Can you work these out from the model? Positions are in its coordinate system, mm. Round coordinates to 2 decimals unless told otherwise and drop trailing zeros. Loops run counter-clockwise (first coordinate to the right, second up) from the corner with the lowest first, then second, coordinate; pieces in that order, holes last.
```python
from build123d import *

# Parameters (mm, degrees)
SKETCH1_R             = 12.7
SKETCH1_R_2           = 2.5
BOSS_EXTRUDE1_DEPTH   = 8.89
F_2_56_TAPPED_HOLE1_D = 1.778
SKETCH6_W             = 1.1303
SKETCH6_H             = 12.7


with BuildPart() as part:
    # Sketch1 → Boss-Extrude1 (new body)
    with BuildSketch(Plane.XY):
        Circle(SKETCH1_R)
        Circle(SKETCH1_R_2, mode=Mode.SUBTRACT)
    extrude(amount=BOSS_EXTRUDE1_DEPTH)

    # #2-56 Tapped Hole1 (through all)
    with Locations(Plane.XY.offset(8.89)):
        with Locations((-8.255, 6.35), (8.255, 6.35), (8.255, -6.35), (-8.255, -6.35)):
            Hole(F_2_56_TAPPED_HOLE1_D / 2)

    # Sketch6 → #4-40 Tapped Hole1 (revolve, cut)
    with BuildSketch(Plane(origin=(0, 0, 4.445), x_dir=(0, 0, -1), z_dir=(1, 0, 0))):
        with Locations((0.56515, 6.35)):
            Rectangle(SKETCH6_W, SKETCH6_H)
    revolve(axis=Axis((0, -6.35, 4.445), (0, 1, 0)), mode=Mode.SUBTRACT)


solid = part.part
```
(1) If I drill on line 1 (Y direction, x = 0, z = 7); line 2 (X direction, y = 6.5, z = 3.25); line 3 (X direction, y = -6, z = 1.75), over which ranges is the centre line in solid material (lowest first)?
(2) We'd pull the mould along Y, two halves only. Please class faces 1 (the cylindrical face through (0.69, 7.54, 5.34)), 2 (the cylindrical face through (-2.75, -12.4, 4.38)), 3 (the cylindrical face through (-0.54, -2.44, 4.38)): released by +Y, released by -Y, zero draft, split by the parting line, or undercut.
(3) Suppose I cut it at B-B (y = 0). Write out the boundary of the cut face in (x, z).
(4) Suppose I cut it at C-C (y = -6.35). Write out the boundary of the cut face in (x, z), then the cut area to 3 significant figures.
(5) Suppose I cut it at D-D (z = 2). Write out the boundary of the cut face in (x, y) (3 decimals).
(6) For pin 1 (1.5 mm diameter, centred on y = 1.5, z = 5.5, fed in from -X); pin 2 (1 mm diameter, centred on x = 6, z = 4.5, fed in from -Y); pin 3 (4 mm diameter, centred on x = 3, z = 1, fed in from -Y), each with a flat end and sliding along its axis, tell me the tip position at first contact or that it passes through.
(7) Suppose I cut it at A-A (x = 0). Write out the boundary of the cut face in (y, z), then the cut area to 3 significant figures.
Check result:
1. line 1: y = -12.7 to -2.5, 2.5 to 12.7
1. line 2: x = -10.91 to -9.13, -7.38 to 7.38, 9.13 to 10.91
1. line 3: x = -11.19 to -9.07, -7.44 to 7.44, 9.07 to 11.19
2. face 1: zero draft
2. face 2: split by the parting line
2. face 3: undercut
3. outline: (-12.7, 0) - (-2.5, 0) - (-2.5, 8.89) - (-12.7, 8.89) - close; (2.5, 0) - (12.7, 0) - (12.7, 8.89) - (2.5, 8.89) - close
4. outline: (-11, 0) - (-9.14, 0) - (-9.14, 8.89) - (-11, 8.89) - close; (-7.37, 0) - (7.37, 0) - (7.37, 8.89) - (-7.37, 8.89) - close; (9.14, 0) - (11, 0) - (11, 8.89) - (9.14, 8.89) - close
4. area: 164 mm2
5. outline: circle Ø25.4 at (0, 0); hole circle Ø1.778 at (-8.255, -6.35); hole circle Ø1.778 at (-8.255, 6.35); hole circle Ø5 at (0, 0); hole circle Ø1.778 at (8.255, -6.35); hole circle Ø1.778 at (8.255, 6.35)
6. pin 1: stops at x = -12.68
6. pin 2: stops at y = -11.45
6. pin 3: stops at y = -12.66
7. outline: (-12.7, 0) - (-2.5, 0) - (-2.5, 8.89) - (-12.7, 8.89) - close; (2.5, 0) - (12.7, 0) - (12.7, 3.31) - (2.5, 3.31) - close; (2.5, 5.58) - (12.7, 5.58) - (12.7, 8.89) - (2.5, 8.89) - close
7. area: 158 mm2
